The listing builds one solid part. Answer for the finished solid, in the listing's coordinates (mm). A direction names the side the tool comes from. Give positions to 0.01 mm unless a question says otherwise; leave off trailing zeros. Write each loop counter-clockwise with the first axis right and the second up, starting at its lowest first coordinate (ties: lowest second). Pieces come first, ordered by that corner, then holes.
```python
from build123d import *

# Parameters (mm, degrees)
SKETCH1_R           = 2.4892
SKETCH1_R_2         = 14.2875
BOSS_EXTRUDE1_DEPTH = 3.175


with BuildPart() as part:
    # Sketch1 → Boss-Extrude1 (new body)
    with BuildSketch(Plane(origin=(0, 0, -3.175), x_dir=(-1, 0, 0), z_dir=(0, 0, -1))):
        with BuildLine():
            Line((8.578679656, -97.553569989), (11.821320344, -94.310929302))
            ThreePointArc((11.821320344, -94.310929302), (12.471638598, -93.337659255), (12.7, -92.189608958))
            Line((12.7, -92.189608958), (12.7, -26.475183996))
            ThreePointArc((12.7, -26.475183996), (13.770167962, -22.947313016), (16.619960204, -20.608548965))
            Line((16.619960204, -20.608548965), (17.010278569, -20.446873805))
            ThreePointArc((17.010278569, -20.446873805), (19.070366834, -19.070366834), (20.446873805, -17.010278569))
            Line((20.446873805, -17.010278569), (26.486206447, -2.430039796))
            ThreePointArc((26.486206447, -2.430039796), (26.969571416, 0), (26.486206447, 2.430039796))
            Line((26.486206447, 2.430039796), (20.446873805, 17.010278569))
            ThreePointArc((20.446873805, 17.010278569), (19.070366834, 19.070366834), (17.010278569, 20.446873805))
            Line((17.010278569, 20.446873805), (2.430039796, 26.486206447))
            ThreePointArc((2.430039796, 26.486206447), (0, 26.969571416), (-2.430039796, 26.486206447))
            Line((-2.430039796, 26.486206447), (-17.010278569, 20.446873805))
            ThreePointArc((-17.010278569, 20.446873805), (-19.070366834, 19.070366834), (-20.446873805, 17.010278569))
            Line((-20.446873805, 17.010278569), (-26.486206447, 2.430039796))
            ThreePointArc((-26.486206447, 2.430039796), (-26.969571416, 0), (-26.486206447, -2.430039796))
            Line((-26.486206447, -2.430039796), (-20.446873805, -17.010278569))
            ThreePointArc((-20.446873805, -17.010278569), (-19.070366834, -19.070366834), (-17.010278569, -20.446873805))
            Line((-17.010278569, -20.446873805), (-16.619960204, -20.608548965))
            ThreePointArc((-16.619960204, -20.608548965), (-13.770167962, -22.947313016), (-12.7, -26.475183996))
            Line((-12.7, -26.475183996), (-12.7, -92.189608958))
            ThreePointArc((-12.7, -92.189608958), (-12.471638598, -93.337659255), (-11.821320344, -94.310929302))
            Line((-11.821320344, -94.310929302), (-8.578679656, -97.553569989))
            ThreePointArc((-8.578679656, -97.553569989), (-7.60540961, -98.203888243), (-6.457359313, -98.432249645))
            Line((-6.457359313, -98.432249645), (6.457359313, -98.432249645))
            ThreePointArc((6.457359313, -98.432249645), (7.60540961, -98.203888243), (8.578679656, -97.553569989))
        make_face()
        with Locations((12.7, -12.7)):
            Circle(SKETCH1_R, mode=Mode.SUBTRACT)
        Circle(SKETCH1_R_2, mode=Mode.SUBTRACT)
        with Locations((-12.7, 12.7)):
            Circle(SKETCH1_R, mode=Mode.SUBTRACT)
        with Locations((-17.960512242, 0)):
            Circle(SKETCH1_R, mode=Mode.SUBTRACT)
        with Locations((-12.7, -12.7)):
            Circle(SKETCH1_R, mode=Mode.SUBTRACT)
        with Locations((12.7, 12.7)):
            Circle(SKETCH1_R, mode=Mode.SUBTRACT)
        with Locations((17.960512242, 0)):
            Circle(SKETCH1_R, mode=Mode.SUBTRACT)
        with Locations((0, 17.960512242)):
            Circle(SKETCH1_R, mode=Mode.SUBTRACT)
        with Locations((0, -22.232249645)):
            Circle(SKETCH1_R, mode=Mode.SUBTRACT)
        with Locations((0, -73.032249645)):
            Circle(SKETCH1_R, mode=Mode.SUBTRACT)
        with Locations((0, -47.632249645)):
            Circle(SKETCH1_R, mode=Mode.SUBTRACT)
        with Locations((0, -34.932249645)):
            Circle(SKETCH1_R, mode=Mode.SUBTRACT)
        with Locations((0, -60.332249645)):
            Circle(SKETCH1_R, mode=Mode.SUBTRACT)
        with Locations((0, -85.732249645)):
            Circle(SKETCH1_R, mode=Mode.SUBTRACT)
    extrude(amount=-BOSS_EXTRUDE1_DEPTH)


solid = part.part
```
Item 1: A cutting plane is placed at A-A, the plane y = -12.7. Give the vertices of the cut face in (x, z) (3 decimals), plus the area to 3 significant figures.
Conclusion:
outline: (-22.232, -3.175) - (-15.189, -3.175) - (-15.189, 0) - (-22.232, 0) - close; (-10.211, -3.175) - (-6.545, -3.175) - (-6.545, 0) - (-10.211, 0) - close; (6.545, -3.175) - (10.211, -3.175) - (10.211, 0) - (6.545, 0) - close; (15.189, -3.175) - (22.232, -3.175) - (22.232, 0) - (15.189, 0) - close
area: 68.0 mm2
Item 2: A cutting plane is placed at C-C, the plane y = -91. Give the vertices of the cut face in (x, z) (3 decimals).
Conclusion:
outline: (-12.7, -3.175) - (12.7, -3.175) - (12.7, 0) - (-12.7, 0) - close
Item 3: Determine the mould class of faces 4 (the face through (0.324, -45.164, -1.61)), 5 (the face through (7.621, -98.198, -1.61)), 6 (the face through (-26.97, -0.03, -1.61)) for opening direction X: pulls with the +X half, pulls with the -X half, needs draft (parallel to the pull), parting line crosses it, or undercut.
Conclusion:
face 4: undercut
face 5: pulls with the +X half
face 6: pulls with the -X half
Item 4: Each of these flat-tipped pins is pushed along its axis until it touches: P1, Ø1, axis at x = -11.5, z = -0.5, coming from the -Y side; P2, Ø4.5, axis at x = 0, y = -60.33, coming from the -Z side; P3, Ø1.5, axis at x = 9.5, z = -2.5, coming from the +Y side; P4, Ø1, axis at y = -40, z = -1.5, coming from the -X side. Where does it stop, or does it pass through?
Conclusion:
P1: stops at y = -95.13
P2: passes through
P3: stops at y = 23.87
P4: stops at x = -12.7
Item 5: Which of the six approach directions +Z, -Z, +X, -X, +Y, -Y give full straight-line access (tool end or side, diameter ignored) to faces 1 (the face through (12.7, -59, -2)), 2 (the face through (9.62, 23.51, -1.61)), 3 (the face through (-12.7, -60, -2))?
Conclusion:
face 1: +Z, -Z, +X, -Y
face 2: +Z, -Z, +X, +Y
face 3: +Z, -Z, -X, -Y
Item 6: A cutting plane is placed at B-B, the plane x = 0. Count the separate pieces of the cut face and the enclosed holes in it, plus the area to 3 significant figures.
Conclusion:
separate pieces: 9
enclosed holes: 0
area: 197 mm2
Item 7: Consider probe 1 along X at (y, z) = (-47, -2.15); probe 2 along X at (y, z) = (-86, -1.4); probe 3 along Y at (x, z) = (17, -0.3). Determine where each line is inside the solid, lowest interval first.
Conclusion:
probe 1: x = -12.7 to -2.41, 2.41 to 12.7
probe 2: x = -12.7 to -2.47, 2.47 to 12.7
probe 3: y = -20.45 to -2.3, 2.3 to 20.45
